```python
from build123d import *

# Parameters (mm, degrees)
PAD001_DEPTH    = 20
SKETCH004_W     = 9
SKETCH004_H     = 6
POCKET001_DEPTH = 8
PAD006_DEPTH    = 50
SKETCH013_W     = 54.5
SKETCH013_H     = 10.071398
PAD007_DEPTH    = 20
SKETCH014_R     = 5
PAD008_DEPTH    = 10
SKETCH015_R     = 3.4
POCKET005_DEPTH = 25
SKETCH016_W     = 54.5
SKETCH016_H     = 5
PAD009_DEPTH    = 40
SKETCH017_W     = 54.5
SKETCH017_H     = 4
PAD010_DEPTH    = 15


with BuildPart() as part:
    # Sketch002 → Pad001 (new body)
    with BuildSketch(Plane.YZ):
        Polygon((-27.098937, -22.548221), (27.401063, -22.548221), (27.401063, 8.451779), (20.651063, 8.451779), (20.651063, -19.548221), (-20.348937, -19.548221), (-20.348937, 8.451779), (-27.098937, 8.451779), align=None)
    extrude(amount=PAD001_DEPTH)

    # Sketch004 → Pocket001 (cut)
    with BuildSketch(Plane(origin=(0, 27.401063, 0), x_dir=(-1, 0, 0), z_dir=(0, 1, 0))):
        with Locations((-9.865053, -13.762334)):
            Rectangle(SKETCH004_W, SKETCH004_H)
    extrude(amount=-POCKET001_DEPTH, mode=Mode.SUBTRACT)

    # Sketch003 (on Face4 of Pocket001) → Pad006 (join)
    with BuildSketch(Plane(origin=(0, 0, 0), x_dir=(0, 1, 0), z_dir=(-1, 0, 0))):
        Polygon((-21.047689, 17.881043), (-26.254499, 17.881043), (-26.254499, 22.454655), (26.951211, 22.454655), (26.951211, 17.881043), (21.744401, 17.881043), (21.744401, 19.754328), (-21.047689, 19.754328), align=None)
    extrude(amount=PAD006_DEPTH)

    # Sketch013 (on Face23 of Pad006) → Pad007 (join)
    with BuildSketch(Plane(origin=(-50, 0, 0), x_dir=(0, 1, 0), z_dir=(-1, 0, 0))):
        with Locations((0.151063, 17.512522)):
            Rectangle(SKETCH013_W, SKETCH013_H)
    extrude(amount=PAD007_DEPTH)

    # Sketch014 (on Face6 of Pad007) → Pad008 (join)
    with BuildSketch(Plane(origin=(0, 0, -12.476823), x_dir=(0, -1, 0), z_dir=(0, 0, 1))):
        with Locations((-0.151063, -60)):
            Circle(SKETCH014_R)
    extrude(amount=PAD008_DEPTH)

    # Sketch015 (on Face17 of Pad008) → Pocket005 (cut)
    with BuildSketch(Plane(origin=(0, 0, -2.476823), x_dir=(0, -1, 0), z_dir=(0, 0, 1))):
        with Locations((-0.151063, -60)):
            Circle(SKETCH015_R)
    extrude(amount=-POCKET005_DEPTH, mode=Mode.SUBTRACT)

    # Sketch016 (on Face27 of Pocket005) → Pad009 (join)
    with BuildSketch(Plane.YZ.offset(20)):
        with Locations((0.151063, -20.048221)):
            Rectangle(SKETCH016_W, SKETCH016_H)
    extrude(amount=PAD009_DEPTH)

    # Sketch017 (on Face37 of Pad009) → Pad010 (join)
    with BuildSketch(Plane(origin=(0, 0, -17.548221), x_dir=(0, -1, 0), z_dir=(0, 0, 1))):
        with Locations((-0.151063, 58)):
            Rectangle(SKETCH017_W, SKETCH017_H)
    extrude(amount=PAD010_DEPTH)


solid = part.part
```
Read the model definition and answer for the solid it produces. Units are mm, in the model's axes. A direction names the side the tool comes from. Round coordinates to 2 decimals unless told otherwise and drop trailing zeros. Loops run counter-clockwise (first coordinate to the right, second up) from the corner with the lowest first, then second, coordinate; pieces in that order, holes last. Notation, with made-up numbers: (70.25, -20) -> (124.25, -20) arc R5 ccw to (124.25, -12) -> close; hole circle Ø3 at (-29, 7.25). An arc over 180 degrees is marked (long way). One line per item, written item: value.
1) The mould has two halves that part along Z. Classify faces 1 (the face through (58, 1, -2.548)), 2 (the face through (10, 24, -16.762)), 3 (the face through (5.365, 24, -14)), 4 (the face through (-70, 0, -18)): pulls with the +Z half, pulls with the -Z half, needs draft (parallel to the pull), parting line crosses it, or undercut.
Answer list:
face 1: pulls with the +Z half
face 2: undercut
face 3: undercut
face 4: needs draft
2) A cutting plane is placed at C-C (z = 0). Determine the outline of the cut face in (x, y), and give its area (3 significant figures).
Answer list:
outline: (0, -27.1) -> (20, -27.1) -> (20, -20.35) -> (0, -20.35) -> close; (0, 20.65) -> (20, 20.65) -> (20, 27.4) -> (0, 27.4) -> close
area: 270 mm²
3) Flat-ended cylindrical pins translate along their axes: P1, Ø5.5, axis at x = -23.5, y = 24.5, coming from the +Z side; P2, Ø25, axis at x = -26, y = -0.5, coming from the -Z side; P3, Ø10, axis at x = -13, y = -1, coming from the +Z side; P4, Ø9.5, axis at y = -3, z = -9.5, coming from the -X side. Find the tip coordinate at first contact, or state that the pin passes through.
Answer list:
P1: stops at z = -17.88
P2: stops at z = -22.45
P3: stops at z = -19.75
P4: stops at x = -70
4) A cutting plane is placed at A-A (z = -8.5). Determine the outline of the cut face in (x, y).
Answer list:
outline: circle Ø10 at (-60, 0.15); (0, -27.1) -> (20, -27.1) -> (20, -20.35) -> (0, -20.35) -> close; (0, 20.65) -> (20, 20.65) -> (20, 27.4) -> (0, 27.4) -> close; (56, -27.1) -> (60, -27.1) -> (60, 27.4) -> (56, 27.4) -> close; hole circle Ø6.8 at (-60, 0.15)
5) A cutting plane is placed at B-B (x = -60). Determine the outline of the cut face in (y, z), and give its area (3 significant figures).
Answer list:
outline: (-27.1, -22.55) -> (-3.25, -22.55) -> (-3.25, -2.48) -> (-4.85, -2.48) -> (-4.85, -12.48) -> (-27.1, -12.48) -> close; (3.55, -22.55) -> (27.4, -22.55) -> (27.4, -12.48) -> (5.15, -12.48) -> (5.15, -2.48) -> (3.55, -2.48) -> close
area: 512 mm²
6) Consider L1, parallel to X at y = 0.5, z = -14; L2, parallel to X at y = -5, z = -13; L3, parallel to Z at x = -32, y = 9.5. Determine where each line is inside the solid, lowest interval first. Write a range as [from, to].
Answer list:
L1: x = [-70, -63.38], [-56.62, -50], [56, 60]
L2: x = [-70, -50], [56, 60]
L3: z = [-22.45, -19.75]
7) For faces 5 (the face through (-25, 0, -22.455)), 6 (the face through (14.365, 24, -14)), 7 (the face through (20, -24, -4)), 8 (the face through (-55.043, 0.802, -7.547)), determine the directions among +Z, -Z, +X, -X, +Y, -Y from which every point of the face is accessible in a straight line to the end or side of a thin tool.
Answer list:
face 5: -Z, +Y, -Y
face 6: +Y
face 7: +Z, +Y, -Y
face 8: +Z
8) A cutting plane is placed at D-D (y = -19). Determine the outline of the cut face in (x, z), and give its area (3 significant figures).
Answer list:
outline: (-70, -22.55) -> (-50, -22.55) -> (-50, -22.45) -> (0, -22.45) -> (0, -22.55) -> (60, -22.55) -> (60, -2.55) -> (56, -2.55) -> (56, -17.55) -> (20, -17.55) -> (20, -19.55) -> (0, -19.55) -> (0, -19.75) -> (-50, -19.75) -> (-50, -12.48) -> (-70, -12.48) -> close
area: 656 mm²
